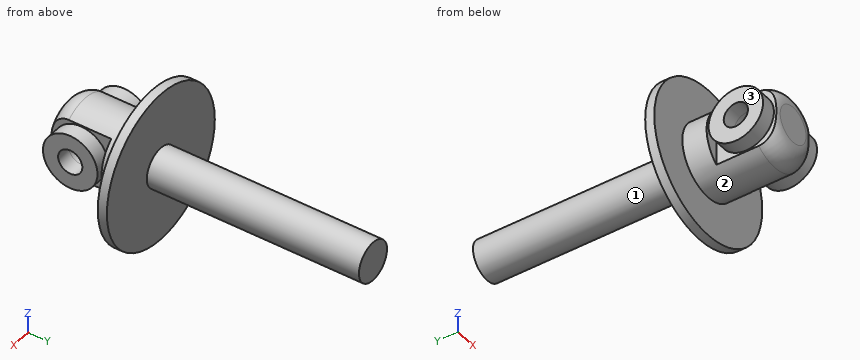
```python
from build123d import *
from build123d.topology import SkipClean

# Parameters (mm, degrees)
SKETCH1_R               = 25
BOSS_EXTRUDE1_DEPTH     = 3
SKETCH2_R               = 6.5
BOSS_EXTRUDE2_DEPTH     = 70
SKETCH3_R               = 12
BOSS_EXTRUDE3_DEPTH     = 28
FILLET1_R               = 6
CUT_EXTRUDE1_DEPTH      = 82.111035008
CUT_EXTRUDE1_DEPTH_BACK = 82.111035008
SKETCH4_W               = 15
SKETCH4_H               = 20
CUT_EXTRUDE2_DEPTH      = 84.727235712
CUT_EXTRUDE2_DEPTH_BACK = 84.727235712
SKETCH5_R               = 4
SKETCH7_R               = 9
SKETCH7_R_2             = 4
BOSS_EXTRUDE4_DEPTH     = 12.5


with BuildPart() as part:
    # Sketch1 → Boss-Extrude1 (new body)
    with BuildSketch(Plane(origin=(0, 0, 0), x_dir=(1, 0, 0), z_dir=(0, 1, 0))):
        with Locations(Location((0, 0, 0), (0, 0, 270))):
            Circle(SKETCH1_R)
    extrude(amount=BOSS_EXTRUDE1_DEPTH)

    # Sketch2 → Boss-Extrude2 (add)
    with BuildSketch(Plane(origin=(0, 3, 0), x_dir=(1, 0, 0), z_dir=(0, 1, 0))):
        with Locations(Location((0, 0, 0), (0, 0, 270))):
            Circle(SKETCH2_R)
    extrude(amount=BOSS_EXTRUDE2_DEPTH)

    # Sketch3 → Boss-Extrude3 (add)
    with BuildSketch(Plane.XZ):
        with Locations(Location((0, 0, 0), (0, 0, 90))):
            Circle(SKETCH3_R)
    extrude(amount=BOSS_EXTRUDE3_DEPTH)

    # Fillet1
    fillet1_edges = [part.edges().sort_by_distance(p)[0] for p in [
        (0, -28, -12),
    ]]
    fillet(fillet1_edges, radius=FILLET1_R)

    # Sketch4 → Cut-Extrude1 (cut, two sides: drawn at the far end of the back side and taken through both)
    with BuildSketch(Plane.XY.offset(-CUT_EXTRUDE1_DEPTH_BACK)):
        with Locations((-15, -18)):
            Rectangle(SKETCH4_W, SKETCH4_H)
        with Locations((15, -18)):
            Rectangle(SKETCH4_W, SKETCH4_H)
    extrude(amount=CUT_EXTRUDE1_DEPTH + CUT_EXTRUDE1_DEPTH_BACK, mode=Mode.SUBTRACT)

    # Sketch5 → Cut-Extrude2 (cut, two sides: drawn at the far end of the back side and taken through both)
    with BuildSketch(Plane(origin=(7.5, 0, 0), x_dir=(0, 0, -1), z_dir=(1, 0, 0)).offset(-CUT_EXTRUDE2_DEPTH_BACK)):
        with Locations(Location((0, -18, 0), (0, 0, 90))):
            Circle(SKETCH5_R)
    extrude(amount=CUT_EXTRUDE2_DEPTH + CUT_EXTRUDE2_DEPTH_BACK, mode=Mode.SUBTRACT)

    # Sketch7 → Boss-Extrude4 (add, symmetric)
    with SkipClean():  # the faces are left unmerged after this step: merging them gives an invalid solid
        with BuildSketch(Plane(origin=(0, 0, 0), x_dir=(0, 0, -1), z_dir=(1, 0, 0))):
            with Locations(Location((0, -18, 0), (0, 0, 90))):
                Circle(SKETCH7_R)
            with Locations((0, -18)):
                Circle(SKETCH7_R_2, mode=Mode.SUBTRACT)
        extrude(amount=BOSS_EXTRUDE4_DEPTH, both=True)


solid = part.part
```
Design review of the part built by this model. Coordinates are the model's own, in mm. Face numbers are marked on the shaded views. A direction names the side the tool comes from. Round coordinates to 2 decimals unless told otherwise and drop trailing zeros. Order: outer loops, then holes, each group sorted by start corner. A loop starts at its lowest first (then second) coordinate and runs counter-clockwise, first axis right, second up. Notation, with made-up numbers: M 19.5,26.5 L 38.5,26.5 A14 ccw 38.5,37.5 Z; hole C 67,-9.75 d3. An arc over 180 degrees is marked long. Put each result on its own line as item: value.
Q1. To check wall thickness, follow line 1 (Z direction, x = -10, y = -18); line 2 (Y direction, x = 3, z = 0); line 3 (Z direction, x = 2.5, y = 46.5). State the ranges of each line that lie inside material, in increasing order.
Reported:
line 1: -9 to -4, 4 to 9
line 2: -28 to -22, -14 to 73
line 3: -6 to 6
Q2. Consider section B-B (y = 60). State the section outline as (x, z) points, and give its area (3 significant figures).
Reported:
outline: C 0,0 d13
area: 133 mm²
Q3. Machinability: for the marked faces 1, 2 and 3, which of the approach directions +Z, -Z, +X, -X, +Y, -Y give a long, thin tool a straight path to every point of the face, cutting with its end or side? Answer none if there is none.
Reported:
face 1: +Y
face 2: none
face 3: +Z, -Z, -X, -Y
Q4. Consider section A-A (z = 15). State the section outline as (x, y) points.
Reported:
outline: M -20,0 L 20,0 L 20,3 L -20,3 Z
Q5. Consider section C-C (x = -20). State the section outline as (y, z) points, and give its area (3 significant figures).
Reported:
outline: M 0,-15 L 3,-15 L 3,15 L 0,15 Z
area: 90.0 mm²
Q6. Insertion check: pin 1 Ø20 at (y, z) = (-18, -1) entering from +X; pin 2 Ø3.5 at (x, z) = (10, -3.5) entering from -Y; pin 3 Ø10 at (y, z) = (34.5, 8) entering from +X. Each pin has a flat end and moves straight along its axis. Give the tip position at first contact, or say it passes through.
Reported:
pin 1: x = 12.5
pin 2: y = -26.83
pin 3: x = 5.77
